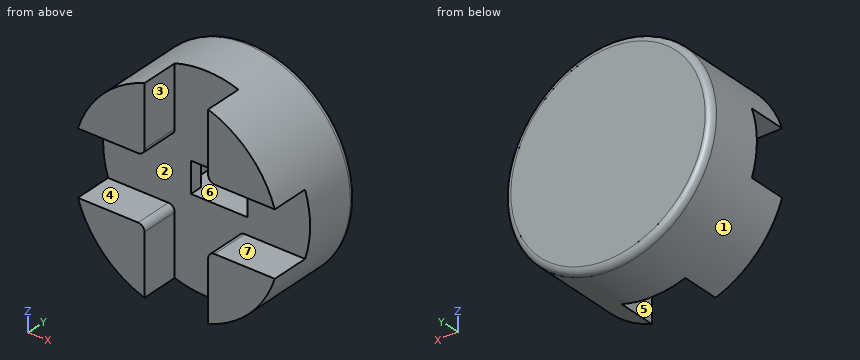
```python
from build123d import *

# Parameters (mm, degrees)
SKETCH2_R           = 41.275
BOSS_EXTRUDE2_DEPTH = 38.1
SKETCH3_R           = 38.735
CUT_EXTRUDE1_DEPTH  = 3.81
SKETCH4_W           = 25.4
SKETCH4_H           = 25.4
CUT_EXTRUDE2_DEPTH  = 15.24
SKETCH5_W           = 32.004
SKETCH5_H           = 12.192
CUT_EXTRUDE3_DEPTH  = 13.97
SKETCH6_W           = 22.606
SKETCH6_H           = 12.192
CUT_EXTRUDE4_DEPTH  = 62.807391548
FILLET1_R           = 2.54


with BuildPart() as part:
    # Sketch2 → Boss-Extrude2 (new body)
    with BuildSketch(Plane(origin=(0, 0, 0), x_dir=(1, 0, 0), z_dir=(0, 1, 0))):
        with Locations(Location((0, 0, 0), (0, 0, 90))):
            Circle(SKETCH2_R)
    extrude(amount=BOSS_EXTRUDE2_DEPTH)

    # Sketch3 → Cut-Extrude1 (cut)
    with BuildSketch(Plane(origin=(0, 38.1, 0), x_dir=(1, 0, 0), z_dir=(0, 1, 0))):
        with Locations(Location((0, 0, 0), (0, 0, 270))):
            Circle(SKETCH3_R)
    extrude(amount=-CUT_EXTRUDE1_DEPTH, mode=Mode.SUBTRACT)

    # Sketch4 → Cut-Extrude2 (cut)
    with BuildSketch(Plane.XZ):
        with BuildLine():
            ThreePointArc((-12.7, -39.272581084), (-6.428446216, -40.771322081), (-6e-08, -41.275))
            ThreePointArc((-6e-08, -41.275), (6.428446158, -40.77132209), (12.7, -39.272581084))
            Line((12.7, -39.272581084), (12.7, -12.7))
            Line((12.7, -12.7), (-12.7, -12.7))
            Line((-12.7, -12.7), (-12.7, -39.272581084))
        make_face()
        Rectangle(SKETCH4_W, SKETCH4_H)
        with BuildLine():
            Line((-12.7, 39.272581084), (-12.7, 12.7))
            Line((-12.7, 12.7), (12.7, 12.7))
            Line((12.7, 12.7), (12.7, 39.272581084))
            ThreePointArc((12.7, 39.272581084), (6.428446095, 40.7713221), (-1.86e-07, 41.275))
            ThreePointArc((-1.86e-07, 41.275), (-6.428446279, 40.771322071), (-12.7, 39.272581084))
        make_face()
        with BuildLine():
            Line((12.7, 12.7), (12.7, -12.7))
            Line((12.7, -12.7), (39.272581084, -12.7))
            ThreePointArc((39.272581084, -12.7), (40.771322086, -6.428446187), (41.275, 0))
            ThreePointArc((41.275, 0), (40.771322086, 6.428446187), (39.272581084, 12.7))
            Line((39.272581084, 12.7), (12.7, 12.7))
        make_face()
        with BuildLine():
            Line((-39.272581084, -12.7), (-12.7, -12.7))
            Line((-12.7, -12.7), (-12.7, 12.7))
            Line((-12.7, 12.7), (-39.272581084, 12.7))
            ThreePointArc((-39.272581084, 12.7), (-40.77132209, 6.428446159), (-41.275, -5.7e-08))
            ThreePointArc((-41.275, -5.7e-08), (-40.771322081, -6.428446215), (-39.272581084, -12.7))
        make_face()
    extrude(amount=-CUT_EXTRUDE2_DEPTH, mode=Mode.SUBTRACT)

    # Sketch5 → Cut-Extrude3 (cut)
    with BuildSketch(Plane(origin=(0, 34.29, 0), x_dir=(1, 0, 0), z_dir=(0, 1, 0))):
        with Locations((5.08, 0)):
            Rectangle(SKETCH5_W, SKETCH5_H)
    extrude(amount=-CUT_EXTRUDE3_DEPTH, mode=Mode.SUBTRACT)

    # Sketch6 → Cut-Extrude4 (cut, through all)
    with BuildSketch(Plane(origin=(0, 20.32, 0), x_dir=(1, 0, 0), z_dir=(0, 1, 0))):
        with Locations((5.08, 0)):
            Rectangle(SKETCH6_W, SKETCH6_H)
    extrude(amount=-CUT_EXTRUDE4_DEPTH, mode=Mode.SUBTRACT)

    # Fillet1
    fillet1_edges = [part.edges().sort_by_distance(p)[0] for p in [
        (12.7, 7.62, 12.7),
        (-12.7, 7.62, 12.7),
        (-12.7, 7.62, -12.7),
        (12.7, 7.62, -12.7),
        (0, 38.1, 41.275),
    ]]
    fillet(fillet1_edges, radius=FILLET1_R - 0.0001)  # a hair under: the kernel refuses the full size


solid = part.part
```
Design review of the part built by this model. Coordinates are the model's own, in mm. Face numbers are marked on the shaded views. A direction names the side the tool comes from. Give positions to 0.01 mm unless a question says otherwise; leave off trailing zeros. Order: outer loops, then holes, each group sorted by start corner. A loop starts at its lowest first (then second) coordinate and runs counter-clockwise, first axis right, second up. Notation, with made-up numbers: (27.25, 57.5) - (68.25, 57.5) arc R15 ccw to (68.25, 70.5) - close; hole circle Ø9 at (86.5, -36.5). An arc over 180 degrees is marked (long way). Use a Markdown table: item, result. Add a question column.
(1) Wall thickness on probe 1 along X at (y, z) = (35, 0) (3 decimals); probe 2 along Y at (x, z) = (6, 26.5); probe 3 along Z at (x, y) = (-8, 25): over which ranges is each line inside the solid? List them lowest first. Write a range as [from, to].
(2) Clearance check with flat-ended pins moving along their axes: P1, Ø3, axis at x = -8, y = 33, coming from the -Z side; P2, Ø1, axis at x = -28, y = 6.5, coming from the -Z side; P3, Ø4.5, axis at y = 9.5, z = -24.5, coming from the +X side. State where each tip first meets the part, or that it passes through.
(3) Mouldability with a two-part tool opening along X and no side actions: class the marked faces 1, 2, 3 and 4 as +X half, -X half, draft (parallel to the pull), parting line (faces both ways), or undercut.
(4) Add section C-C on y = 22. Give the boundary of the cut face in (x, z) (3 decimals).
(5) Machinability: for the marked faces 5, 6 and 7, which of the approach directions +Z, -Z, +X, -X, +Y, -Y give a long, thin tool a straight path to every point of the face, cutting with its end or side? Answer none if there is none.
Report:
| question | item | result |
|---|---|---|
| 1 | probe 1 | x = [-41.275, -38.735], [38.735, 41.275] |
| 1 | probe 2 | y = [15.24, 34.29] |
| 1 | probe 3 | z = [-40.49, -6.1], [6.1, 40.49] |
| 2 | P1 | stops at z = -40.76 |
| 2 | P2 | stops at z = -30.78 |
| 2 | P3 | stops at x = 34.76 |
| 3 | face 1 | parting line |
| 3 | face 2 | undercut |
| 3 | face 3 | undercut |
| 3 | face 4 | draft |
| 4 | outline | circle Ø82.55 at (0, 0); hole (-10.922, -6.096) - (21.082, -6.096) - (21.082, 6.096) - (-10.922, 6.096) - close |
| 5 | face 5 | +Z, -Z, -Y |
| 5 | face 6 | +Y |
| 5 | face 7 | +X, -X, -Y |
